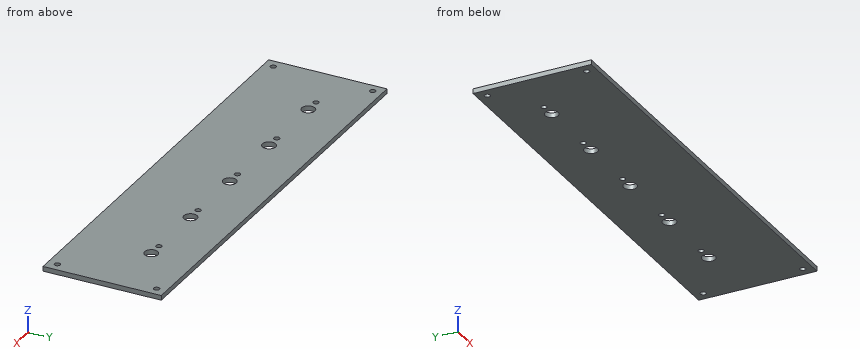
```python
from build123d import *

# Parameters (mm, degrees)
SKETCH1_W           = 230
SKETCH1_H           = 62.43
BOSS_EXTRUDE1_DEPTH = 2.5
SKETCH2_R           = 1.5
CUT_EXTRUDE1_DEPTH  = 10
SKETCH3_R           = 3.5
SKETCH3_R_2         = 1.5
CUT_EXTRUDE2_DEPTH  = 2.5


with BuildPart() as part:
    # Sketch1 → Boss-Extrude1 (new body)
    with BuildSketch(Plane.XY):
        with Locations((115, 31.215)):
            Rectangle(SKETCH1_W, SKETCH1_H)
    extrude(amount=BOSS_EXTRUDE1_DEPTH)

    # Sketch2 → Cut-Extrude1 (cut)
    with BuildSketch(Plane.XY.offset(2.5)):
        with Locations((5, 57.43)):
            Circle(SKETCH2_R)
        with Locations((5, 5)):
            Circle(SKETCH2_R)
        with Locations((225, 5)):
            Circle(SKETCH2_R)
        with Locations((225, 57.43)):
            Circle(SKETCH2_R)
    extrude(amount=-CUT_EXTRUDE1_DEPTH, mode=Mode.SUBTRACT)

    # Sketch3 → Cut-Extrude2 (cut)
    with BuildSketch(Plane.XY.offset(2.5)):
        with Locations((115, 39.01875)):
            Circle(SKETCH3_R)
        with Locations((107.2, 39.01875)):
            Circle(SKETCH3_R_2)
        with Locations((155, 39.01875)):
            Circle(SKETCH3_R)
        with Locations((147.2, 39.01875)):
            Circle(SKETCH3_R_2)
        with Locations((195, 39.01875)):
            Circle(SKETCH3_R)
        with Locations((187.2, 39.01875)):
            Circle(SKETCH3_R_2)
        with Locations((67.2, 39.01875)):
            Circle(SKETCH3_R_2)
        with Locations((75, 39.01875)):
            Circle(SKETCH3_R)
        with Locations((27.2, 39.01875)):
            Circle(SKETCH3_R_2)
        with Locations((35, 39.01875)):
            Circle(SKETCH3_R)
    extrude(amount=-CUT_EXTRUDE2_DEPTH, mode=Mode.SUBTRACT)


solid = part.part
```
The model under review builds one solid part; all positions refer to its coordinate system, in mm. Round coordinates to 2 decimals unless told otherwise and drop trailing zeros. Loops run counter-clockwise (first coordinate to the right, second up) from the corner with the lowest first, then second, coordinate; pieces in that order, holes last.
Item 1: Take a section at B-B (z = 0.5). Give the number of separate pieces and of enclosed holes in the cut face, then the cut area to 3 significant figures.
Determined:
separate pieces: 1
enclosed holes: 14
area: 14,100 mm2
Item 2: Take a section at A-A (x = 35). Write out the cut boundary in (y, z).
Determined:
outline: (0, 0) - (35.52, 0) - (35.52, 2.5) - (0, 2.5) - close; (42.52, 0) - (62.43, 0) - (62.43, 2.5) - (42.52, 2.5) - close
Item 3: For line 1 (Y direction, x = 5, z = 2.05); line 2 (Y direction, x = 115, z = 0.5); line 3 (X direction, y = 56.5, z = 1.9), list the stretches that pass through material, from the lowest coordinate up.
Determined:
line 1: y = 0 to 3.5, 6.5 to 55.93, 58.93 to 62.43
line 2: y = 0 to 35.52, 42.52 to 62.43
line 3: x = 0 to 3.82, 6.18 to 223.82, 226.18 to 230
Item 4: Clearance check with a flat-ended pin moving along its axis: pin 1 Ø2.5 at (x, y) = (107.2, 39.02) entering from -Z. State where the tip first meets the part, or that it passes through.
Determined:
pin 1: passes through
